For this review, take the finished solid that the model builds, in its own axes (mm). A direction names the side the tool comes from. Give positions to 0.01 mm unless a question says otherwise; leave off trailing zeros. Write each loop counter-clockwise with the first axis right and the second up, starting at its lowest first coordinate (ties: lowest second). Pieces come first, ordered by that corner, then holes.
1) We need section D-D on x = -28. Give the boundary of the cut face in (y, z), and give its area (3 significant figures).
2) Machinability: for faces 1 (the face through (0, 1, -35)), 2 (the face through (19.5, 1, -38)), which of the approach directions +Z, -Z, +X, -X, +Y, -Y give a long, thin tool a straight path to every point of the face, cutting with its end or side? Answer none if there is none.
3) We need section A-A on y = 0.25. Give the boundary of the cut face in (x, z), and give its area (3 significant figures).
4) We need section B-B on x = 17.5. Give the boundary of the cut face in (y, z), and give its area (3 significant figures).
5) We need section C-C on z = -37.75. Give the boundary of the cut face in (x, y).
6) Draft analysis for pull direction X (two halves, no side actions). For faces 3 (the face through (-19.5, 1, -38)), 4 (the face through (0, 0, -40)), 5 (the face through (0.506, 0.74, -47.997)), state which applies: pulls with the +X half, pulls with the -X half, needs draft (parallel to the pull), parting line crosses it, or undercut.
7) Wall thickness on line 1 along Z through (x, y) = (0.5, 0.1); line 2 along Z through (x, y) = (-5, 0.65); line 3 along X through (y, z) = (0.45, -38): over which ranges is each line inside the solid? List them lowest first.
from build123d import *

# Parameters (mm, degrees)
SKETCH1_R           = 48
BOSS_EXTRUDE1_DEPTH = 1.5
CUT_EXTRUDE1_START  = -1.5
CUT_EXTRUDE1_DEPTH  = 1.5
SKETCH3_W           = 39
SKETCH3_H           = 1.8
CUT_EXTRUDE2_DEPTH  = 1.5


with BuildPart() as part:
    # Sketch1 → Boss-Extrude1 (new body)
    with BuildSketch(Plane(origin=(0, 0, 0), x_dir=(1, 0, 0), z_dir=(0, 1, 0))):
        with Locations(Location((0, 0, 0), (0, 0, 270))):
            Circle(SKETCH1_R)
    extrude(amount=BOSS_EXTRUDE1_DEPTH)

    # Sketch2 → Cut-Extrude1 (cut)
    with BuildSketch(Plane(origin=(0, 1.5, 0), x_dir=(1, 0, 0), z_dir=(0, 1, 0)).offset(CUT_EXTRUDE1_START)):
        with BuildLine():
            Line((-32.848135411, 35), (32.848135411, 35))
            ThreePointArc((32.848135411, 35), (0, -48), (-32.848135411, 35))
        make_face()
    extrude(amount=CUT_EXTRUDE1_DEPTH, mode=Mode.SUBTRACT)

    # Sketch3 → Cut-Extrude2 (cut)
    with BuildSketch(Plane(origin=(0, 1.5, 0), x_dir=(1, 0, 0), z_dir=(0, 1, 0))):
        with Locations((0, 37.9)):
            Rectangle(SKETCH3_W, SKETCH3_H)
    extrude(amount=-CUT_EXTRUDE2_DEPTH, mode=Mode.SUBTRACT)


solid = part.part
Results list:
1. outline: (0, -38.99) - (1.5, -38.99) - (1.5, -35) - (0, -35) - close
1. area: 5.98 mm2
2. face 1: +Z, +X, -X, +Y, -Y
2. face 2: +Y, -Y
3. outline: (-32.85, -35) arc R48 ccw to (32.85, -35) - close; hole (-19.5, -38.8) - (19.5, -38.8) - (19.5, -37) - (-19.5, -37) - close
3. area: 517 mm2
4. outline: (0, -44.7) - (1.5, -44.7) - (1.5, -38.8) - (0, -38.8) - close; (0, -37) - (1.5, -37) - (1.5, -35) - (0, -35) - close
4. area: 11.8 mm2
5. outline: (-29.65, 0) - (-19.5, 0) - (-19.5, 1.5) - (-29.65, 1.5) - close; (19.5, 0) - (29.65, 0) - (29.65, 1.5) - (19.5, 1.5) - close
6. face 3: undercut
6. face 4: needs draft
6. face 5: parting line crosses it
7. line 1: z = -48 to -38.8, -37 to -35
7. line 2: z = -47.74 to -38.8, -37 to -35
7. line 3: x = -29.33 to -19.5, 19.5 to 29.33
